Geometry: see drawing. Coordinates: mm, zero at the bounding-box minimum. Give positions to 0.01 mm unless a question says otherwise; leave off trailing zeros. Write each loop counter-clockwise with the first axis right and the second up, starting at its lowest first coordinate (ties: lowest second). Pieces come first, ordered by that corner, then holes. Notation, with made-up numbers: (20, 21) - (25, 21) arc R28 ccw to (25, 41) - close; hole circle Ø1 at (68, 69.5). An arc over 180 degrees is marked (long way). Use CSV: the item, a comma, the result in double quotes. Start each with the question number.
(1) Section A-A on y = 86. Output: boundary loops of the cut face in (x, z) (3 decimals), and give its area (3 significant figures).
(2) Line query: probe 1 along Y at (x, z) = (86, 6.75) (3 decimals); probe 2 along X at (y, z) = (63.5, 1.5). Output: solid intervals per line, ascending. Write a range as [from, to].
(3) First-contact query: pin 1 Ø2 at (x, y) = (86, 86) entering from -Z. Flat tip, straight axial feed; report the tip coordinate or a pass-through.
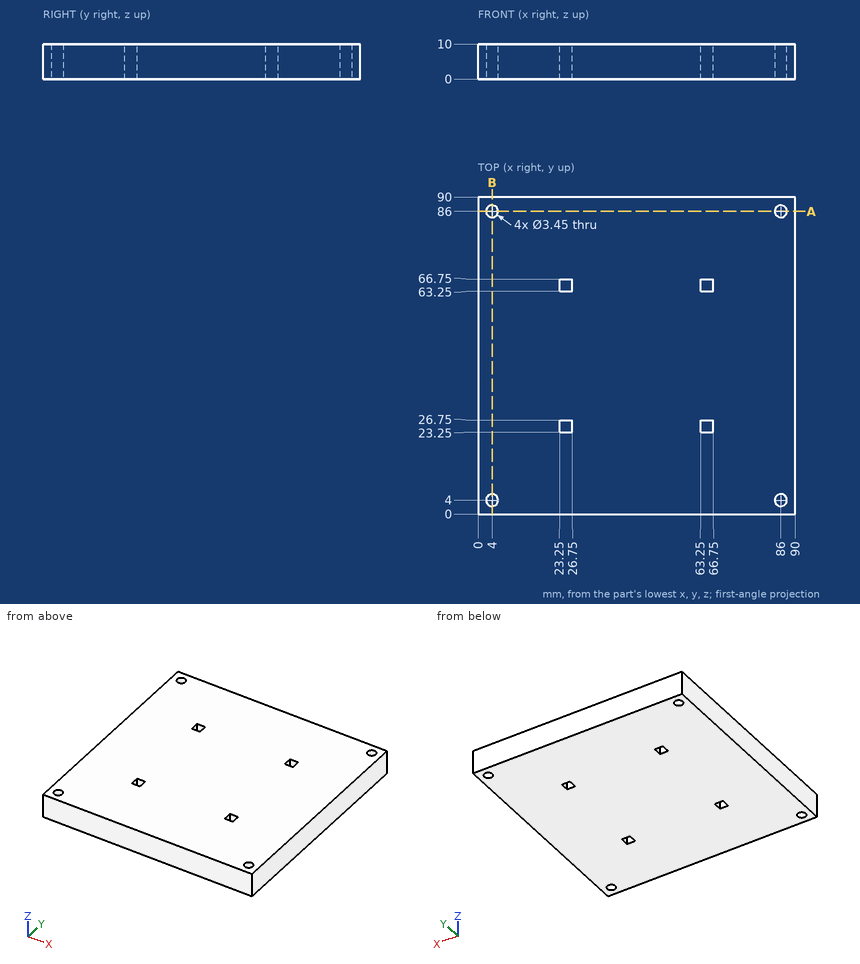
Check values:
1,outline,"(0, 0) - (2.275, 0) - (2.275, 10) - (0, 10) - close; (5.725, 0) - (84.275, 0) - (84.275, 10) - (5.725, 10) - close; (87.725, 0) - (90, 0) - (90, 10) - (87.725, 10) - close"
1,area,"831 mm²"
2,probe 1,"y = [0, 2.275], [5.725, 84.275], [87.725, 90]"
2,probe 2,"x = [0, 23.25], [26.75, 63.25], [66.75, 90]"
3,pin 1,"passes through"
